Input: part model. Units: mm. Frame: model coordinates. Coordinates: 2 decimals unless noted, no trailing zeros. Write each loop counter-clockwise with the first axis right and the second up, starting at its lowest first coordinate (ties: lowest second). Pieces come first, ordered by that corner, then holes. Notation, with made-up numbers: (9, 7.5) - (67, 7.5) arc R8 cw to (67, 11.5) - close; hole circle Ø8 at (13, 38). An arc over 180 degrees is marked (long way). Use a Markdown table: item, result. Add a question column.
Q1. Pin query (flat end, axial travel): P1, Ø1.5, axis at x = 1201.5, z = 2, coming from the -Y side; P2, Ø1.5, axis at x = 910, z = 3, coming from the +Y side; P3, Ø1.5, axis at x = 66, z = 1.5, coming from the -Y side. Return the tip coordinate at first contact, or that it passes through.
Q2. Section query B-B (z = 2.25). Give the number of separate pieces and of enclosed holes in the cut face, then the cut area to 3 significant figures.
Q3. Section query A-A (x = 756). Return the cut outline in (y, z).
Q4. Material intervals for probe 1 along Y at (x, z) = (799.5, 3.7); probe 2 along Y at (x, z) = (502, 1.55); probe 3 along Y at (x, z) = (1165, 3), sorted ascending. Write a range as from..to.
from build123d import *

# Parameters (mm, degrees)
BOSS_EXTRUDE1_DEPTH     = 5.08
CUT_EXTRUDE4_DEPTH      = 6.08
SKETCH1_4_R             = 9.398
CUT_EXTRUDE7_DEPTH      = 6.08
CUT_EXTRUDE7_DEPTH_BACK = 1


with BuildPart() as part:
    # Sketch1 → Boss-Extrude1 (new body)
    with BuildSketch(Plane.XY):
        with BuildLine():
            Line((0, 0), (12.898944119, 0))
            ThreePointArc((12.898944119, 0), (16.172901968, -1.195724006), (17.905619663, -4.22))
            ThreePointArc((17.905619663, -4.22), (25.6159, -10.7188), (33.326180337, -4.22))
            ThreePointArc((33.326180337, -4.22), (35.058898032, -1.195724006), (38.332855881, 0))
            Line((38.332855881, 0), (111.450944119, 0))
            ThreePointArc((111.450944119, 0), (114.724901968, -1.195724006), (116.457619663, -4.22))
            ThreePointArc((116.457619663, -4.22), (124.1679, -10.7188), (131.878180337, -4.22))
            ThreePointArc((131.878180337, -4.22), (133.610898032, -1.195724006), (136.884855881, 0))
            Line((136.884855881, 0), (210.002944119, 0))
            ThreePointArc((210.002944119, 0), (213.276901968, -1.195724006), (215.009619663, -4.22))
            ThreePointArc((215.009619663, -4.22), (222.7199, -10.7188), (230.430180337, -4.22))
            ThreePointArc((230.430180337, -4.22), (232.162898032, -1.195724006), (235.436855881, 0))
            Line((235.436855881, 0), (308.554944119, 0))
            ThreePointArc((308.554944119, 0), (311.828901968, -1.195724006), (313.561619663, -4.22))
            ThreePointArc((313.561619663, -4.22), (321.2719, -10.7188), (328.982180337, -4.22))
            ThreePointArc((328.982180337, -4.22), (330.714898032, -1.195724006), (333.988855881, 0))
            Line((333.988855881, 0), (407.106944119, 0))
            ThreePointArc((407.106944119, 0), (410.380901968, -1.195724006), (412.113619663, -4.22))
            ThreePointArc((412.113619663, -4.22), (419.8239, -10.7188), (427.534180337, -4.22))
            ThreePointArc((427.534180337, -4.22), (429.266898032, -1.195724006), (432.540855881, 0))
            Line((432.540855881, 0), (505.658944119, 0))
            ThreePointArc((505.658944119, 0), (508.932901968, -1.195724006), (510.665619663, -4.22))
            ThreePointArc((510.665619663, -4.22), (518.3759, -10.7188), (526.086180337, -4.22))
            ThreePointArc((526.086180337, -4.22), (527.818898032, -1.195724006), (531.092855881, 0))
            Line((531.092855881, 0), (604.210944119, 0))
            ThreePointArc((604.210944119, 0), (607.484901968, -1.195724006), (609.217619663, -4.22))
            ThreePointArc((609.217619663, -4.22), (616.9279, -10.7188), (624.638180337, -4.22))
            ThreePointArc((624.638180337, -4.22), (626.370898032, -1.195724006), (629.644855881, 0))
            Line((629.644855881, 0), (702.762944119, 0))
            ThreePointArc((702.762944119, 0), (706.036901968, -1.195724006), (707.769619663, -4.22))
            ThreePointArc((707.769619663, -4.22), (715.4799, -10.7188), (723.190180337, -4.22))
            ThreePointArc((723.190180337, -4.22), (724.922898032, -1.195724006), (728.196855881, 0))
            Line((728.196855881, 0), (801.314944119, 0))
            ThreePointArc((801.314944119, 0), (804.588901968, -1.195724006), (806.321619663, -4.22))
            ThreePointArc((806.321619663, -4.22), (814.0319, -10.7188), (821.742180337, -4.22))
            ThreePointArc((821.742180337, -4.22), (823.474898032, -1.195724006), (826.748855881, 0))
            Line((826.748855881, 0), (899.866944119, 0))
            ThreePointArc((899.866944119, 0), (903.140901968, -1.195724006), (904.873619663, -4.22))
            ThreePointArc((904.873619663, -4.22), (912.5839, -10.7188), (920.294180337, -4.22))
            ThreePointArc((920.294180337, -4.22), (922.026898032, -1.195724006), (925.300855881, 0))
            Line((925.300855881, 0), (998.418944119, 0))
            ThreePointArc((998.418944119, 0), (1001.692901968, -1.195724006), (1003.425619663, -4.22))
            ThreePointArc((1003.425619663, -4.22), (1011.1359, -10.7188), (1018.846180337, -4.22))
            ThreePointArc((1018.846180337, -4.22), (1020.578898032, -1.195724006), (1023.852855881, 0))
            Line((1023.852855881, 0), (1096.970944119, 0))
            ThreePointArc((1096.970944119, 0), (1100.244901968, -1.195724006), (1101.977619663, -4.22))
            ThreePointArc((1101.977619663, -4.22), (1109.6879, -10.7188), (1117.398180337, -4.22))
            ThreePointArc((1117.398180337, -4.22), (1119.130898032, -1.195724006), (1122.404855881, 0))
            Line((1122.404855881, 0), (1195.522944119, 0))
            ThreePointArc((1195.522944119, 0), (1198.796901968, -1.195724006), (1200.529619663, -4.22))
            ThreePointArc((1200.529619663, -4.22), (1208.2399, -10.7188), (1215.950180337, -4.22))
            ThreePointArc((1215.950180337, -4.22), (1217.682898032, -1.195724006), (1220.956855881, 0))
            Line((1220.956855881, 0), (1294.074944119, 0))
            ThreePointArc((1294.074944119, 0), (1297.348901968, -1.195724006), (1299.081619663, -4.22))
            ThreePointArc((1299.081619663, -4.22), (1306.7919, -10.7188), (1314.502180337, -4.22))
            ThreePointArc((1314.502180337, -4.22), (1316.234898032, -1.195724006), (1319.508855881, 0))
            Line((1319.508855881, 0), (1353.185, 0))
            Line((1353.185, 0), (1353.185, -8.6614))
            Line((1353.185, -8.6614), (1373.0986, -29.4894))
            Line((1373.0986, -29.4894), (1396.1364, -29.4894))
            Line((1396.1364, -29.4894), (1416.05, -12.7762))
            Line((1416.05, -12.7762), (1416.05, 15.367))
            Line((1416.05, 15.367), (1397.95671204, 42.671885143))
            ThreePointArc((1397.95671204, 42.671885143), (1385.175201607, 49.825078541), (1371.926438397, 43.57964356))
            Line((1371.926438397, 43.57964356), (1353.185, 19.177))
            Line((1353.185, 19.177), (0, 19.177))
            Line((0, 19.177), (0, 0))
        make_face()
    extrude(amount=BOSS_EXTRUDE1_DEPTH)

    # Sketch2 → Cut-Extrude4 (cut, through all)
    with BuildSketch(Plane.XY.offset(5.08)):
        with BuildLine():
            Line((9.7409, 15.9512), (41.4909, 15.9512))
            ThreePointArc((41.4909, 15.9512), (44.6659, 12.7762), (41.4909, 9.6012))
            Line((41.4909, 9.6012), (9.7409, 9.6012))
            ThreePointArc((9.7409, 9.6012), (6.5659, 12.7762), (9.7409, 15.9512))
        make_face()
        with BuildLine():
            Line((108.2929, 15.9512), (140.0429, 15.9512))
            ThreePointArc((140.0429, 15.9512), (143.2179, 12.7762), (140.0429, 9.6012))
            Line((140.0429, 9.6012), (108.2929, 9.6012))
            ThreePointArc((108.2929, 9.6012), (105.1179, 12.7762), (108.2929, 15.9512))
        make_face()
        with BuildLine():
            Line((206.8449, 15.9512), (238.5949, 15.9512))
            ThreePointArc((238.5949, 15.9512), (241.7699, 12.7762), (238.5949, 9.6012))
            Line((238.5949, 9.6012), (206.8449, 9.6012))
            ThreePointArc((206.8449, 9.6012), (203.6699, 12.7762), (206.8449, 15.9512))
        make_face()
        with BuildLine():
            Line((305.3969, 15.9512), (337.1469, 15.9512))
            ThreePointArc((337.1469, 15.9512), (340.3219, 12.7762), (337.1469, 9.6012))
            Line((337.1469, 9.6012), (305.3969, 9.6012))
            ThreePointArc((305.3969, 9.6012), (302.2219, 12.7762), (305.3969, 15.9512))
        make_face()
        with BuildLine():
            Line((403.9489, 15.9512), (435.6989, 15.9512))
            ThreePointArc((435.6989, 15.9512), (438.8739, 12.7762), (435.6989, 9.6012))
            Line((435.6989, 9.6012), (403.9489, 9.6012))
            ThreePointArc((403.9489, 9.6012), (400.7739, 12.7762), (403.9489, 15.9512))
        make_face()
        with BuildLine():
            Line((502.5009, 15.9512), (534.2509, 15.9512))
            ThreePointArc((534.2509, 15.9512), (537.4259, 12.7762), (534.2509, 9.6012))
            Line((534.2509, 9.6012), (502.5009, 9.6012))
            ThreePointArc((502.5009, 9.6012), (499.3259, 12.7762), (502.5009, 15.9512))
        make_face()
        with BuildLine():
            Line((601.0529, 15.9512), (632.8029, 15.9512))
            ThreePointArc((632.8029, 15.9512), (635.9779, 12.7762), (632.8029, 9.6012))
            Line((632.8029, 9.6012), (601.0529, 9.6012))
            ThreePointArc((601.0529, 9.6012), (597.8779, 12.7762), (601.0529, 15.9512))
        make_face()
        with BuildLine():
            Line((699.6049, 15.9512), (731.3549, 15.9512))
            ThreePointArc((731.3549, 15.9512), (734.5299, 12.7762), (731.3549, 9.6012))
            Line((731.3549, 9.6012), (699.6049, 9.6012))
            ThreePointArc((699.6049, 9.6012), (696.4299, 12.7762), (699.6049, 15.9512))
        make_face()
        with BuildLine():
            Line((798.1569, 15.9512), (829.9069, 15.9512))
            ThreePointArc((829.9069, 15.9512), (833.0819, 12.7762), (829.9069, 9.6012))
            Line((829.9069, 9.6012), (798.1569, 9.6012))
            ThreePointArc((798.1569, 9.6012), (794.9819, 12.7762), (798.1569, 15.9512))
        make_face()
        with BuildLine():
            Line((896.7089, 15.9512), (928.4589, 15.9512))
            ThreePointArc((928.4589, 15.9512), (931.6339, 12.7762), (928.4589, 9.6012))
            Line((928.4589, 9.6012), (896.7089, 9.6012))
            ThreePointArc((896.7089, 9.6012), (893.5339, 12.7762), (896.7089, 15.9512))
        make_face()
        with BuildLine():
            Line((995.2609, 15.9512), (1027.0109, 15.9512))
            ThreePointArc((1027.0109, 15.9512), (1030.1859, 12.7762), (1027.0109, 9.6012))
            Line((1027.0109, 9.6012), (995.2609, 9.6012))
            ThreePointArc((995.2609, 9.6012), (992.0859, 12.7762), (995.2609, 15.9512))
        make_face()
        with BuildLine():
            Line((1093.8129, 15.9512), (1125.5629, 15.9512))
            ThreePointArc((1125.5629, 15.9512), (1128.7379, 12.7762), (1125.5629, 9.6012))
            Line((1125.5629, 9.6012), (1093.8129, 9.6012))
            ThreePointArc((1093.8129, 9.6012), (1090.6379, 12.7762), (1093.8129, 15.9512))
        make_face()
        with BuildLine():
            Line((1192.3649, 15.9512), (1224.1149, 15.9512))
            ThreePointArc((1224.1149, 15.9512), (1227.2899, 12.7762), (1224.1149, 9.6012))
            Line((1224.1149, 9.6012), (1192.3649, 9.6012))
            ThreePointArc((1192.3649, 9.6012), (1189.1899, 12.7762), (1192.3649, 15.9512))
        make_face()
        with BuildLine():
            Line((1290.9169, 15.9512), (1322.6669, 15.9512))
            ThreePointArc((1322.6669, 15.9512), (1325.8419, 12.7762), (1322.6669, 9.6012))
            Line((1322.6669, 9.6012), (1290.9169, 9.6012))
            ThreePointArc((1290.9169, 9.6012), (1287.7419, 12.7762), (1290.9169, 15.9512))
        make_face()
    extrude(amount=-CUT_EXTRUDE4_DEPTH, mode=Mode.SUBTRACT)

    # Sketch1<4> → Cut-Extrude7 (cut, two sides)
    with BuildSketch(Plane.XY) as cut_extrude7_sk:
        with Locations((1384.6175, 33.8328)):
            Circle(SKETCH1_4_R)
    extrude(amount=CUT_EXTRUDE7_DEPTH, mode=Mode.SUBTRACT)
    extrude(cut_extrude7_sk.sketch, amount=-CUT_EXTRUDE7_DEPTH_BACK, mode=Mode.SUBTRACT)


solid = part.part
Values follow:
| question | item | result |
|---|---|---|
| 1 | P1 | y = -7.93 |
| 1 | P2 | y = 19.18 |
| 1 | P3 | y = 0 |
| 2 | separate pieces | 1 |
| 2 | enclosed holes | 15 |
| 2 | area | 28,400 mm2 |
| 3 | outline | (0, 0) - (19.18, 0) - (19.18, 5.08) - (0, 5.08) - close |
| 4 | probe 1 | 0..9.6, 15.95..19.18 |
| 4 | probe 2 | 0..9.64, 15.91..19.18 |
| 4 | probe 3 | 0..19.18 |
